Input: dimensioned drawing with shaded views. Units: mm. Origin: part minimum x, y, z. Coordinates: 2 decimals unless noted, no trailing zeros. Order: outer loops, then holes, each group sorted by start corner. A loop starts at its lowest first (then second) coordinate and runs counter-clockwise, first axis right, second up. Notation, with made-up numbers: (24, 9) -> (43, 9) arc R31 ccw to (43, 41) -> close; hole circle Ø7 at (-31, 16). An arc over 180 degrees is marked (long way). Answer as CSV lines item,"result".
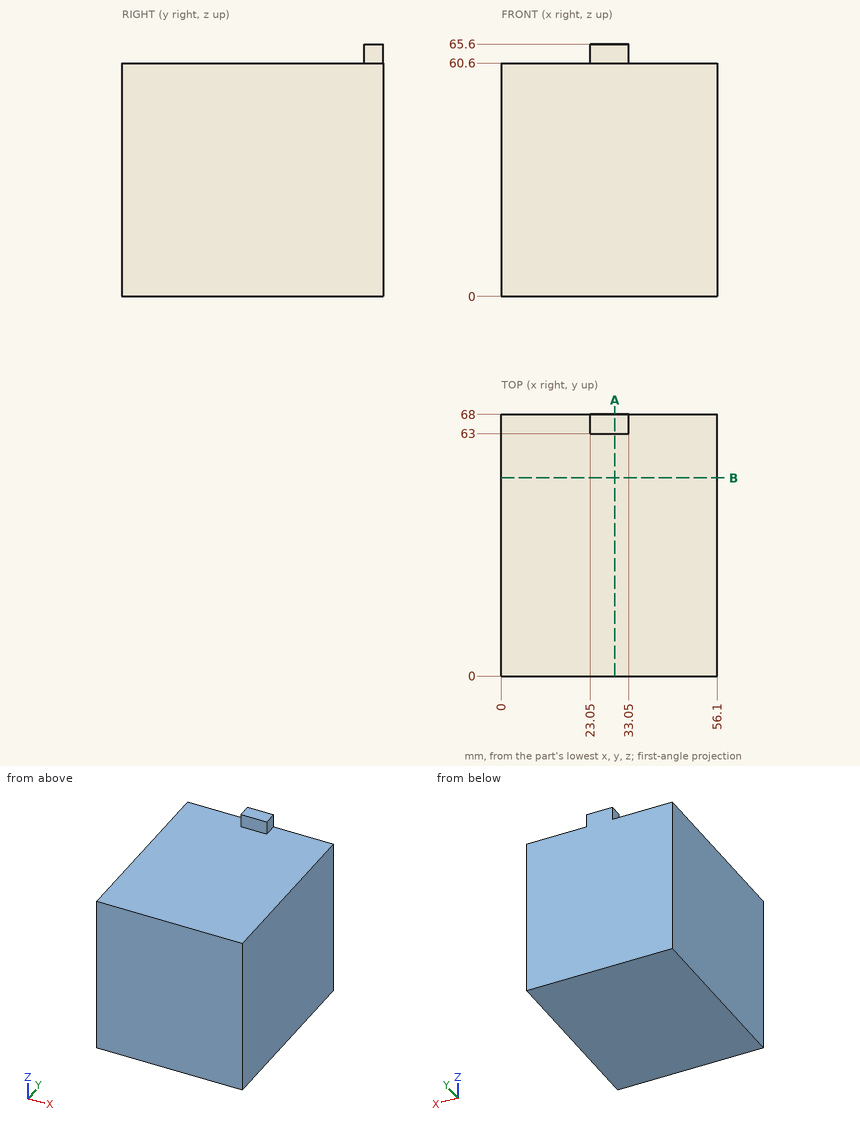
1. Cut plane A-A (x = 29.5). Return the cut outline in (y, z), plus the area to 3 significant figures.
Findings:
outline,"(0, 0) -> (68, 0) -> (68, 65.6) -> (63, 65.6) -> (63, 60.6) -> (0, 60.6) -> close"
area,"4,150 mm2"
2. Ray query, line 1 along Z through (x, y) = (7, 34). Return the intervals inside material, ascending.
Findings:
line 1,"z = 0 to 60.6"
3. Cut plane B-B (y = 51.5). Return the cut outline in (x, z), plus the area to 3 significant figures.
Findings:
outline,"(0, 0) -> (56.1, 0) -> (56.1, 60.6) -> (0, 60.6) -> close"
area,"3,400 mm2"
4. Contact query for flat-ended pins moving along their axis: pin 1 (5.5 mm diameter, centred on y = 65.5, z = 63, fed in from -X); pin 2 (17 mm diameter, centred on x = 14.5, y = 20, fed in from +Z); pin 3 (1.5 mm diameter, centred on x = 25.5, z = 64.5, fed in from -Y). Output: stop coordinate, or through.
Findings:
pin 1,"stops at x = 0"
pin 2,"stops at z = 60.6"
pin 3,"stops at y = 63"
